Check sheet for the modelled part. Datum: model origin and axes. Units: mm. A direction names the side the tool comes from. Round coordinates to 2 decimals unless told otherwise and drop trailing zeros. Write each loop counter-clockwise with the first axis right and the second up, starting at its lowest first coordinate (ties: lowest second). Pieces come first, ordered by that corner, then holes. Notation, with made-up numbers: (-1, -38) -> (30, -38) arc R13 ccw to (30, -25) -> close; hole circle Ø4 at (-8.5, 72). An arc over 180 degrees is marked (long way). One line per item, written item: value. Start each with the question number.
Autodesk Fusion 360 part; units mm, degrees
sketch "Sketch1" plane through (0, 0, 0) normal (0, 0, 1) x (1, 0, 0)
  line L0 (-76.2, 38.1) -> (76.2, 38.1)
  line L1 (76.2, 38.1) -> (76.2, -38.1)
  line L2 (76.2, -38.1) -> (-76.2, -38.1)
  line L3 (-76.2, -38.1) -> (-76.2, 38.1)
  dimension "d1" = 152.4
  dimension "d2" = 76.2
  dimension "d3" = 76.2
  dimension "d4" = 38.1
extrude "Extrude1" add sketch "Sketch1" along normal blind 6.35
sketch "Sketch2" plane through (0, 0, 6.35) normal (0, 0, 1) x (-1, 0, 0)
  line L0 (76.2, 38.1) -> (-76.2, 38.1)
  line L1 (-76.2, 38.1) -> (-76.2, -38.1)
  line L2 (-76.2, -38.1) -> (76.2, -38.1)
  line L3 (76.2, -38.1) -> (76.2, 38.1)
  line L4 (76.2, 38.1) -> (50.8, 38.1)
  line L5 (50.8, 38.1) -> (50.8, 31.75)
  line L6 (50.8, 31.75) -> (76.2, 31.75)
  line L7 (76.2, 31.75) -> (76.2, 38.1)
  line L8 (-76.2, 38.1) -> (-50.8, 38.1)
  line L9 (-50.8, 38.1) -> (-50.8, 31.75)
  line L10 (-50.8, 31.75) -> (-76.2, 31.75)
  line L11 (-76.2, 31.75) -> (-76.2, 38.1)
  line L12 (25.4, 38.1) -> (-25.4, 38.1)
  line L13 (-25.4, 38.1) -> (-25.4, 31.75)
  line L14 (-25.4, 31.75) -> (25.4, 31.75)
  line L15 (25.4, 31.75) -> (25.4, 38.1)
  dimension "d7" = 25.4
  dimension "d8" = 6.35
  dimension "d9" = 25.4
  dimension "d10" = 6.35
  dimension "d11" = 25.4
  dimension "d12" = 25.4
  dimension "d13" = 6.35
extrude "Extrude2" cut sketch "Sketch2" against normal through all contours L0 L3 L4 L5 L6 L7 | L0 L12 L13 L14 L15 | L0 L1 L8 L9 L10 L11
1. Cross-section at B-B (x = 16). Record the cut outline in (y, z), plus the area to 3 significant figures.
2. Cross-section at A-A (z = 3.5). Record the cut outline in (x, y), plus the area to 3 significant figures.
3. Material ranges on probe 1 along Y at (x, z) = (65, 3.75); probe 2 along X at (y, z) = (-33.5, 2.5), recorded low to high.
4. Depth check by flat-ended pin: pin 1 Ø3 at (y, z) = (-35.5, 3.5) entering from +X; pin 2 Ø3 at (y, z) = (-36, 3.5) entering from -X; pin 3 Ø5 at (x, y) = (-8, 28) entering from -Z; pin 4 Ø3 at (x, z) = (-57.5, 2) entering from -Y. Enter the tip coordinate at first touch or a pass-through.
5. Access from +Z, -Z, +X, -X, +Y, -Y to the whole of each face (thin tool, end or side, straight path). Record for faces 1 (the face through (-25.4, -35, 3)), 2 (the face through (50.8, -35, 3)), 3 (the face through (76.2, 4, 3)), 4 (the face through (-63, -31.75, 3)).
Working result:
1. outline: (-31.75, 0) -> (38.1, 0) -> (38.1, 6.35) -> (-31.75, 6.35) -> close
1. area: 444 mm^2
2. outline: (-76.2, -31.75) -> (-50.8, -31.75) -> (-50.8, -38.1) -> (-25.4, -38.1) -> (-25.4, -31.75) -> (25.4, -31.75) -> (25.4, -38.1) -> (50.8, -38.1) -> (50.8, -31.75) -> (76.2, -31.75) -> (76.2, 38.1) -> (-76.2, 38.1) -> close
2. area: 11,000 mm^2
3. probe 1: y = -31.75 to 38.1
3. probe 2: x = -50.8 to -25.4, 25.4 to 50.8
4. pin 1: stops at x = 50.8
4. pin 2: stops at x = -50.8
4. pin 3: stops at z = 0
4. pin 4: stops at y = -31.75
5. face 1: +Z, -Z, -Y
5. face 2: +Z, -Z, +X, -Y
5. face 3: +Z, -Z, +X, +Y, -Y
5. face 4: +Z, -Z, -X, -Y
